Autodesk Inventor part; units mm, degrees
ref_plane "YZ Plane" through (0, 0, 0) normal (1, 0, 0) x (0, 1, 0)
ref_plane "XZ Plane" through (0, 0, 0) normal (0, 1, 0) x (-1, 0, 0)
ref_plane "XY Plane" through (0, 0, 0) normal (0, 0, 1) x (1, 0, 0)
sketch "Sketch1" plane through (0, 0, 0) normal (0, 1, 0) x (-1, 0, 0)
  circle A0 centre (0, 0) radius 6
  dimension "d0" = 12
extrude "Extrusion1" add sketch "Sketch1" along normal blind 150
thread "Thread1"
chamfer "Chamfer1" distance 1 angle 45 1 edges at (6, 150, 0)
fillet "Fillet1" radius 5 1 edges at (6, 0, 0)
properties part number "Griff"
The listing builds one solid part. Answer for the finished solid, in the listing's coordinates (mm). Coordinates: 2 decimals unless noted, no trailing zeros. Write each loop counter-clockwise with the first axis right and the second up, starting at its lowest first coordinate (ties: lowest second). Pieces come first, ordered by that corner, then holes. Notation, with made-up numbers: (56, 21.5) - (61, 21.5) arc R27 cw to (61, 58.5) - close; hole circle Ø5 at (14, 17). An arc over 180 degrees is marked (long way). Return JSON: item names as keys, results as strings. Group by question number.
1. Given pin 1 (1 mm diameter, centred on x = -1, y = 15, fed in from +Z); pin 2 (4 mm diameter, centred on x = -3, z = -1.5, fed in from -Y); pin 3 (1.5 mm diameter, centred on x = 1, z = -4, fed in from -Y), each flat-ended and moving along its own axis, determine where each tip first touches the part or whether it passes through.
2. A cutting plane is placed at A-A, the plane y = 104.5. Determine the outline of the cut face in (x, z), plus the area to 3 significant figures.
3. Straight lines are drawn through the part: L1, parallel to X at y = 122, z = 0.25; L2, parallel to Y at x = -1.25, z = -0.25; L3, parallel to X at y = 70, z = -2.25. For each, find the intervals that lie inside material, in ascending order.
Ans:
{
 "1": {"pin 1": "z = 5.98", "pin 2": "y = 0.01", "pin 3": "y = 0.6"},
 "2": {"outline": "circle Ø12 at (0, 0)", "area": "113 mm²"},
 "3": {"L1": "-5.99 to 5.99", "L2": "0.01 to 150", "L3": "-5.56 to 5.56"}
}
